The listing builds one solid part. Answer for the finished solid, in the listing's coordinates (mm). A direction names the side the tool comes from. Give positions to 0.01 mm unless a question says otherwise; leave off trailing zeros. Write each loop counter-clockwise with the first axis right and the second up, starting at its lowest first coordinate (ties: lowest second). Pieces come first, ordered by that corner, then holes. Notation, with made-up numbers: (83, -27) - (126, -27) arc R19 ccw to (126, -11) - close; hole circle Ø10 at (59.5, 36.25). An arc over 180 degrees is marked (long way). Return JSON: item names as keys, results as strings.
from build123d import *

# Parameters (mm, degrees)
F0_R     = 3
F1_DEPTH = 1
F2_DEPTH = 3
F3_DEPTH = 4


with BuildPart() as f1:
    # F0 (on Top) → F1 (new body)
    with BuildSketch(Plane.XY):
        with BuildLine():
            Line((60, -31.7542648054), (60, 31.7542648054))
            ThreePointArc((60, 31.7542648054), (59.3301270189, 34.2542648054), (57.5, 36.0843918244))
            Line((57.5, 36.0843918244), (2.5, 67.8386566298))
            ThreePointArc((2.5, 67.8386566298), (0, 68.5085296109), (-2.5, 67.8386566298))
            Line((-2.5, 67.8386566298), (-57.5, 36.0843918244))
            ThreePointArc((-57.5, 36.0843918244), (-59.3301270189, 34.2542648054), (-60, 31.7542648054))
            Line((-60, 31.7542648054), (-60, -31.7542648054))
            ThreePointArc((-60, -31.7542648054), (-59.3301270189, -34.2542648054), (-57.5, -36.0843918244))
            Line((-57.5, -36.0843918244), (-2.5, -67.8386566298))
            ThreePointArc((-2.5, -67.8386566298), (0, -68.5085296109), (2.5, -67.8386566298))
            Line((2.5, -67.8386566298), (57.5, -36.0843918244))
            ThreePointArc((57.5, -36.0843918244), (59.3301270189, -34.2542648054), (60, -31.7542648054))
        make_face()
        with Locations((-55.7296181053, -32.1755099552)):
            Circle(F0_R, mode=Mode.SUBTRACT)
        with BuildLine():
            Line((-48.2098294683, -37.1204850669), (-49.760809999, -35.8324663113))
            ThreePointArc((-49.760809999, -35.8324663113), (-49.667440276, -28.6755099601), (-55.9122311458, -25.1778923265))
            Line((-55.9122311458, -25.1778923265), (-56.2521978402, -23.1906944078))
            ThreePointArc((-56.2521978402, -23.1906944078), (-47.9353894676, -27.6755099615), (-48.2098294683, -37.1204850669))
        make_face(mode=Mode.SUBTRACT)
        with Locations((0, -64.35102)):
            Circle(F0_R, mode=Mode.SUBTRACT)
        with BuildLine():
            Line((8.042368383, -60.3111795587), (6.1514211554, -61.0103587227))
            ThreePointArc((6.1514211554, -61.0103587227), (0, -57.35102), (-6.1514211554, -61.0103587227))
            Line((-6.1514211554, -61.0103587227), (-8.042368383, -60.3111795587))
            ThreePointArc((-8.042368383, -60.3111795587), (0, -55.35102), (8.042368383, -60.3111795587))
        make_face(mode=Mode.SUBTRACT)
        with BuildLine():
            Line((56.2521977284, -23.190694679), (55.9122310244, -25.1778925961))
            ThreePointArc((55.9122310244, -25.1778925961), (49.6674401378, -28.6755101995), (49.7608098263, -35.8324665512))
            Line((49.7608098263, -35.8324665512), (48.2098292894, -37.1204852993))
            ThreePointArc((48.2098292894, -37.1204852993), (47.9353893342, -27.6755101926), (56.2521977284, -23.190694679))
        make_face(mode=Mode.SUBTRACT)
        with Locations((55.7296179502, -32.1755102239)):
            Circle(F0_R, mode=Mode.SUBTRACT)
        with Locations((-55.7296180277, 32.1755100895)):
            Circle(F0_R, mode=Mode.SUBTRACT)
        with BuildLine():
            Line((-56.2521977843, 23.1906945434), (-55.9122310851, 25.1778924613))
            ThreePointArc((-55.9122310851, 25.1778924613), (-49.6674402069, 28.6755100798), (-49.7608099126, 35.8324664312))
            Line((-49.7608099126, 35.8324664312), (-48.2098293788, 37.1204851831))
            ThreePointArc((-48.2098293788, 37.1204851831), (-47.9353894009, 27.675510077), (-56.2521977843, 23.1906945434))
        make_face(mode=Mode.SUBTRACT)
        with BuildLine():
            Line((48.2098295578, 37.1204849507), (49.7608100854, 35.8324661914))
            ThreePointArc((49.7608100854, 35.8324661914), (49.6674403451, 28.6755098404), (55.9122312065, 25.1778921918))
            Line((55.9122312065, 25.1778921918), (56.2521978961, 23.1906942723))
            ThreePointArc((56.2521978961, 23.1906942723), (47.9353895343, 27.675509846), (48.2098295578, 37.1204849507))
        make_face(mode=Mode.SUBTRACT)
        with Locations((55.7296181828, 32.1755098209)):
            Circle(F0_R, mode=Mode.SUBTRACT)
        with BuildLine():
            Line((-8.0423682377, 60.311179578), (-6.1514210083, 61.0103587375))
            ThreePointArc((-6.1514210083, 61.0103587375), (1.382e-07, 57.35102), (6.1514213024, 61.0103587079))
            Line((6.1514213024, 61.0103587079), (8.0423685284, 60.3111795393))
            ThreePointArc((8.0423685284, 60.3111795393), (1.334e-07, 55.35102), (-8.0423682377, 60.311179578))
        make_face(mode=Mode.SUBTRACT)
        with Locations((1.551e-07, 64.35102)):
            Circle(F0_R, mode=Mode.SUBTRACT)
    extrude(amount=F1_DEPTH)

    # F0 (on Top) → F2 (join)
    with BuildSketch(Plane.XY):
        with BuildLine():
            ThreePointArc((-6.1514211554, -61.0103587227), (0, -57.35102), (6.1514211554, -61.0103587227))
            Line((6.1514211554, -61.0103587227), (8.042368383, -60.3111795587))
            ThreePointArc((8.042368383, -60.3111795587), (0, -55.35102), (-8.042368383, -60.3111795587))
            Line((-8.042368383, -60.3111795587), (-6.1514211554, -61.0103587227))
        make_face()
        with BuildLine():
            ThreePointArc((-55.9122311458, -25.1778923265), (-49.667440276, -28.6755099601), (-49.760809999, -35.8324663113))
            Line((-49.760809999, -35.8324663113), (-48.2098294683, -37.1204850669))
            ThreePointArc((-48.2098294683, -37.1204850669), (-47.9353894676, -27.6755099615), (-56.2521978402, -23.1906944078))
            Line((-56.2521978402, -23.1906944078), (-55.9122311458, -25.1778923265))
        make_face()
        with BuildLine():
            ThreePointArc((49.7608098263, -35.8324665512), (49.6674401378, -28.6755101995), (55.9122310244, -25.1778925961))
            Line((55.9122310244, -25.1778925961), (56.2521977284, -23.190694679))
            ThreePointArc((56.2521977284, -23.190694679), (47.9353893342, -27.6755101926), (48.2098292894, -37.1204852993))
            Line((48.2098292894, -37.1204852993), (49.7608098263, -35.8324665512))
        make_face()
        with BuildLine():
            ThreePointArc((-49.7608099126, 35.8324664312), (-49.6674402069, 28.6755100798), (-55.9122310851, 25.1778924613))
            Line((-55.9122310851, 25.1778924613), (-56.2521977843, 23.1906945434))
            ThreePointArc((-56.2521977843, 23.1906945434), (-47.9353894009, 27.675510077), (-48.2098293788, 37.1204851831))
            Line((-48.2098293788, 37.1204851831), (-49.7608099126, 35.8324664312))
        make_face()
        with BuildLine():
            ThreePointArc((6.1514213024, 61.0103587079), (1.382e-07, 57.35102), (-6.1514210083, 61.0103587375))
            Line((-6.1514210083, 61.0103587375), (-8.0423682377, 60.311179578))
            ThreePointArc((-8.0423682377, 60.311179578), (1.334e-07, 55.35102), (8.0423685284, 60.3111795393))
            Line((8.0423685284, 60.3111795393), (6.1514213024, 61.0103587079))
        make_face()
        with BuildLine():
            ThreePointArc((55.9122312065, 25.1778921918), (49.6674403451, 28.6755098404), (49.7608100854, 35.8324661914))
            Line((49.7608100854, 35.8324661914), (48.2098295578, 37.1204849507))
            ThreePointArc((48.2098295578, 37.1204849507), (47.9353895343, 27.675509846), (56.2521978961, 23.1906942723))
            Line((56.2521978961, 23.1906942723), (55.9122312065, 25.1778921918))
        make_face()
    extrude(amount=F2_DEPTH)

    # F0 (on Top) → F3 (join)
    with BuildSketch(Plane.XY):
        with Locations((-55.7296181053, -32.1755099552)):
            Circle(F0_R)
        with Locations((0, -64.35102)):
            Circle(F0_R)
        with Locations((55.7296179502, -32.1755102239)):
            Circle(F0_R)
        with Locations((55.7296181828, 32.1755098209)):
            Circle(F0_R)
        with Locations((1.551e-07, 64.35102)):
            Circle(F0_R)
        with Locations((-55.7296180277, 32.1755100895)):
            Circle(F0_R)
    extrude(amount=F3_DEPTH)


solid = f1.part
Item 1: For faces 1 (the face through (-30.38, -51.74, 0.49)), 2 (the face through (58.59, 33.08, 2.48)), determine the directions among +Z, -Z, +X, -X, +Y, -Y from which every point of the face is accessible in a straight line to the end or side of a thin tool.
Answer below:
{"face 1": "+Z, -Z, -X, -Y", "face 2": "+Z"}
Item 2: Consider L1, parallel to X at y = -32.5, z = 2.85; L2, parallel to X at y = -30, z = 1.1; L3, parallel to Z at x = -14.5, y = -10.5. Determine where each line is inside the solid, lowest interval first.
Answer below:
{"L1": "x = -58.71 to -52.75, -48.74 to -46.74, 46.74 to 48.74, 52.75 to 58.71", "L2": "x = -57.8 to -53.66, -49.08 to -47, 47 to 49.08, 53.66 to 57.8", "L3": "z = 0 to 1"}
Item 3: The mould has two halves that part along Y. Classify faces 3 (the face through (56, -32, 4)), 4 (the face through (-49, -29, 3)), 5 (the face through (29.62, -52.18, 0.49)): +Y half, -Y half, draft (parallel to the pull), parting line (faces both ways), or undercut.
Answer below:
{"face 3": "draft", "face 4": "undercut", "face 5": "-Y half"}
Item 4: A cutting plane is placed at C-C on x = 33. Determine the outline of the cut face in (y, z).
Answer below:
{"outline": "(-50.23, 0) - (50.23, 0) - (50.23, 1) - (-50.23, 1) - close"}
Item 5: A cutting plane is placed at B-B on y = 7. Determine the outline of the cut face in (x, z), then the cut area to 3 significant figures.
Answer below:
{"outline": "(-60, 0) - (60, 0) - (60, 1) - (-60, 1) - close", "area": "120 mm²"}
Item 6: Flat-ended cylindrical pins translate along their axes: P1, Ø6, axis at x = 3.5, y = 59, coming from the +Z side; P2, Ø1.5, axis at y = 47.5, z = 3, coming from the +X side; P3, Ø2, axis at y = 31, z = 2.5, coming from the +X side; P4, Ø12, axis at x = 40, y = -42.5, coming from the +Z side. Find the tip coordinate at first contact, or state that the pin passes through.
Answer below:
{"P1": "stops at z = 3", "P2": "passes through", "P3": "stops at x = 58.72", "P4": "stops at z = 1"}
Item 7: A cutting plane is placed at A-A on x = 0. Determine the outline of the cut face in (y, z), then the cut area to 3 significant figures.
Answer below:
{"outline": "(-68.51, 0) - (68.51, 0) - (68.51, 1) - (67.35, 1) - (67.35, 4) - (61.35, 4) - (61.35, 1) - (57.35, 1) - (57.35, 3) - (55.35, 3) - (55.35, 1) - (-55.35, 1) - (-55.35, 3) - (-57.35, 3) - (-57.35, 1) - (-61.35, 1) - (-61.35, 4) - (-67.35, 4) - (-67.35, 1) - (-68.51, 1) - close", "area": "181 mm²"}
